The model under review builds one solid part; all positions refer to its coordinate system, in mm. A direction names the side the tool comes from. Coordinates: 2 decimals unless noted, no trailing zeros. Loops run counter-clockwise (first coordinate to the right, second up) from the corner with the lowest first, then second, coordinate; pieces in that order, holes last. Notation, with made-up numbers: M 2,-23.75 L 53,-23.75 A20 cw 53,-14.75 Z; hole C 26,-9 d8. An arc over 180 degrees is marked long. Return JSON: item names as keys, results as strings.
```python
from build123d import *

# Parameters (mm, degrees)
BOSS_EXTRUDE1_DEPTH     = 2
SKETCH2_W               = 10
SKETCH2_H               = 3
BOSS_EXTRUDE2_DEPTH     = 8
FILLET1_R               = 4
CUT_EXTRUDE1_DEPTH      = 134.747858576
CUT_EXTRUDE1_DEPTH_BACK = 134.747858576
SKETCH3_R               = 1.75


with BuildPart() as part:
    # Sketch1 → Boss-Extrude1 (new body)
    with BuildSketch(Plane(origin=(0, 0, 0), x_dir=(0, 0, -1), z_dir=(1, 0, 0))):
        with BuildLine():
            Line((-40.736833925, 130), (-29.353634228, 130))
            ThreePointArc((-29.353634228, 130), (-4.909489029, 76.705560779), (10, 20))
            Line((10, 20), (10, 0))
            Line((10, 0), (0, 0))
            Line((0, 0), (0, 20))
            ThreePointArc((0, 20), (-15.436156632, 76.826587909), (-40.736833925, 130))
        make_face()
    extrude(amount=BOSS_EXTRUDE1_DEPTH)

    # Sketch2 → Boss-Extrude2 (add)
    with BuildSketch(Plane(origin=(2, 0, 0), x_dir=(0, 0, -1), z_dir=(1, 0, 0))):
        with Locations((5, 1.5)):
            Rectangle(SKETCH2_W, SKETCH2_H)
        with BuildLine():
            Line((-40.736833925, 130), (-29.353634228, 130))
            ThreePointArc((-29.353634228, 130), (-28.507977965, 128.502132743), (-27.669921848, 127))
            Line((-27.669921848, 127), (-38.985998837, 127))
            ThreePointArc((-38.985998837, 127), (-39.857464817, 128.502306179), (-40.736833925, 130))
        make_face()
    extrude(amount=BOSS_EXTRUDE2_DEPTH)

    # Fillet1
    fillet1_edges = [part.edges().sort_by_distance(p)[0] for p in [
        (10, 1.5, 0),
        (10, 1.5, -10),
        (10, 128.502306179, 39.857464817),
        (10, 128.502132743, 28.507977965),
    ]]
    fillet(fillet1_edges, radius=FILLET1_R)

    # Sketch3 → Cut-Extrude1 (cut, two sides: drawn at the far end of the back side and taken through both)
    with BuildSketch(Plane(origin=(0, 3, 0), x_dir=(1, 0, 0), z_dir=(0, 1, 0)).offset(-CUT_EXTRUDE1_DEPTH_BACK)):
        with Locations(Location((6, 5, 0), (0, 0, 270))):
            Circle(SKETCH3_R)
        with Locations(Location((6, -35.031677414, 0), (0, 0, 270))):
            Circle(SKETCH3_R)
    extrude(amount=CUT_EXTRUDE1_DEPTH + CUT_EXTRUDE1_DEPTH_BACK, mode=Mode.SUBTRACT)


solid = part.part
```
1. Add section B-B on z = 9.5. Give the boundary of the cut face in (x, y).
Check values:
{"outline": "M 0,59.3 L 2,59.3 L 2,88.8 L 0,88.8 Z"}
2. Add section A-A on y = 34.5. Give the boundary of the cut face in (x, z).
Check values:
{"outline": "M 0,-7.18 L 2,-7.18 L 2,2.91 L 0,2.91 Z"}
3. To check wall thickness, follow line 1 (X direction, y = 2, z = -5); line 2 (Y direction, x = 9.25, z = 37); line 3 (X direction, y = 35.5, z = -3.5). State the ranges of each line that lie inside material, in increasing order.
Check values:
{"line 1": "0 to 4.25, 7.75 to 10", "line 2": "127 to 130", "line 3": "0 to 2"}
4. The part is to be moulded in two halves that separate along X. For faces 1 (the face through (4.45, 128.48, 35.84)), 2 (the face through (6, 127, 33)), 3 (the face through (0, 65, 6)), 4 (the face through (8.797, 1.521, -1.141)), say which applies: released by +X, released by -X, zero draft, split by the parting line, or undercut.
Check values:
{"face 1": "undercut", "face 2": "zero draft", "face 3": "released by -X", "face 4": "released by +X"}
5. Machinability: for faces 5 (the face through (4, 3, -5)), 6 (the face through (1.6, 7.6, 0)), 7 (the face through (3.97, 128.52, 28.52)), which of the approach directions +Z, -Z, +X, -X, +Y, -Y give a long, thin tool a straight path to every point of the face, cutting with its end or side? Answer none if there is none.
Check values:
{"face 5": "+Z, -Z, +X, +Y", "face 6": "+Z, +X, -X, -Y", "face 7": "-Z, +X, -X, +Y"}
6. Insertion check: pin 1 Ø6 at (x, z) = (2.5, 18.5) entering from +Y; pin 2 Ø4 at (x, z) = (5, -6) entering from +Y; pin 3 Ø12 at (y, z) = (41.5, 7.5) entering from -X; pin 4 Ø2.5 at (x, z) = (5.5, 36) entering from -Y. Each pin has a flat end and moves straight along its axis. Give the tip position at first contact, or say it passes through.
Check values:
{"pin 1": "y = 115.26", "pin 2": "y = 3", "pin 3": "x = 0", "pin 4": "y = 127"}
